Check sheet for the drawn part. Datum: minimum x, y, z corner. Units: mm. A direction names the side the tool comes from. Coordinates: 2 decimals unless noted, no trailing zeros. Loops run counter-clockwise (first coordinate to the right, second up) from the corner with the lowest first, then second, coordinate; pieces in that order, holes last.
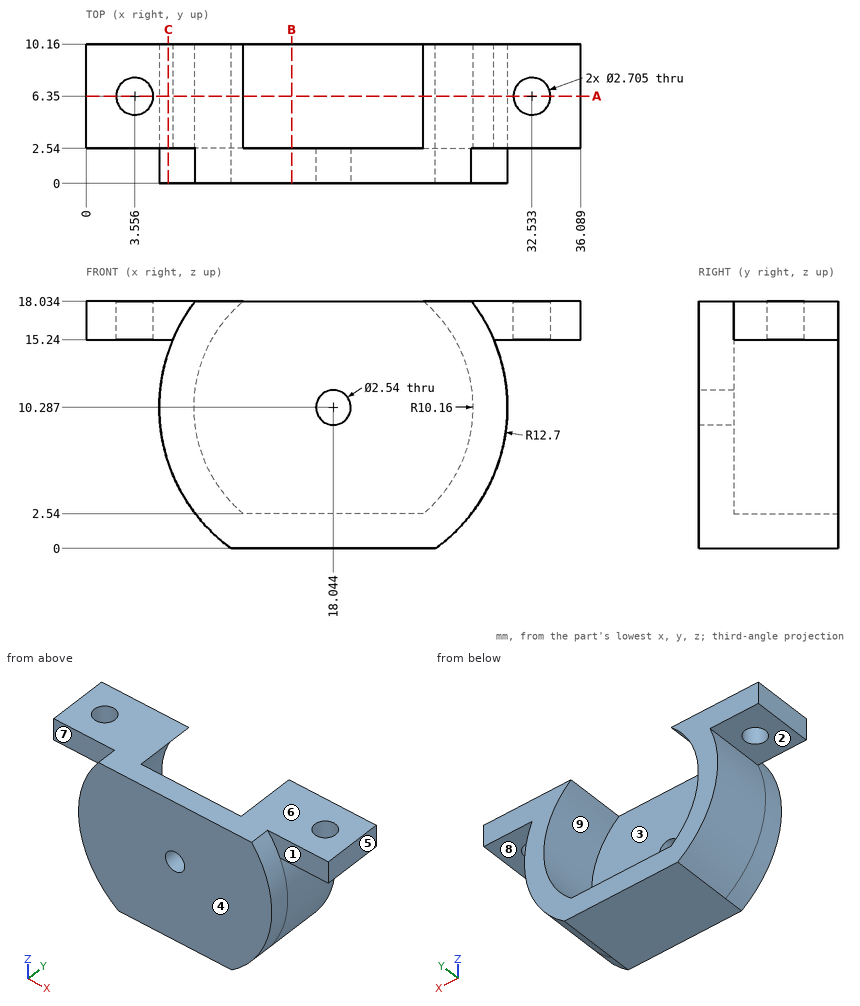
(1) Sectioned sample at C-C on x = 6. Record the cut outline in (y, z) (1 decimal), and give its area (3 significant figures).
Findings:
outline: (0, 6.3) - (10.2, 6.3) - (10.2, 14.3) - (0, 14.3) - close; (2.5, 15.2) - (10.2, 15.2) - (10.2, 18) - (2.5, 18) - close
area: 103 mm2
(2) Access from +Z, -Z, +X, -X, +Y, -Y to the whole of each face (thin tool, end or side, straight path). Record for the marked faces 1, 2, 3, 4 and 5.
Findings:
face 1: +Z, +X, -Y
face 2: -X, +Y, -Y
face 3: +Y
face 4: +Z, -Z, +X, -X, -Y
face 5: +Z, -Z, +X, +Y, -Y
(3) Gauge pin test, flat ends, axial feed: pin 1 Ø2.5 at (x, y) = (20.5, 7.5) entering from +Z; pin 2 Ø5 at (y, z) = (8.5, 10.5) entering from -X; pin 3 Ø6 at (y, z) = (8.5, 2) entering from +X. Record the tip position at first contact, or that the pin passes through.
Findings:
pin 1: stops at z = 2.54
pin 2: stops at x = 5.34
pin 3: stops at x = 29.59
(4) Scan lines: L1, parallel to Y at x = 25.5, z = 12.75; L2, parallel to Z at x = 2, y = 2.75. Record each from-to range of solid material in increasing order.
Findings:
L1: y = 0 to 2.54
L2: z = 15.24 to 18.03
(5) Sectioned sample at A-A on y = 6.35. State how many separate pieces and enclosed holes the cut face has, and give its area (3 significant figures).
Findings:
separate pieces: 3
enclosed holes: 0
area: 156 mm2
(6) Draft check along Z on the marked faces 6, 7, 8 and 9. Enter one of: +Z half, -Z half, draft (parallel to the pull), parting line (faces both ways), or undercut.
Findings:
face 6: +Z half
face 7: draft
face 8: undercut
face 9: undercut
(7) Sectioned sample at B-B on x = 15. Record the cut outline in (y, z).
Findings:
outline: (0, 0) - (10.16, 0) - (10.16, 2.54) - (2.54, 2.54) - (2.54, 18.03) - (0, 18.03) - close
